Here's how the part is built. I have some questions about the finished solid (model axes, mm). Face numbers are marked on the shaded views. A direction names the side the tool comes from. Give positions to 0.01 mm unless a question says otherwise; leave off trailing zeros. Write each loop counter-clockwise with the first axis right and the second up, starting at its lowest first coordinate (ties: lowest second). Pieces come first, ordered by that corner, then holes. Notation, with made-up numbers: (7, 3) -> (64, 3) arc R24 ccw to (64, 21) -> close; hole circle Ø6 at (27, 52). An arc over 180 degrees is marked (long way). Use CSV: the item, a comma, the result in double quotes. Start each with the question number.
(1) For pin 1 Ø5 at (x, y) = (-24, -3.5) entering from +Z; pin 2 Ø0.9 at (y, z) = (0, 2.5) entering from -X; pin 3 Ø2 at (y, z) = (-2, 11.5) entering from -X, each with a flat end and sliding along its axis, tell me the tip position at first contact or that it passes through.
(2) Suppose I cut it at C-C on z = 11. List the corners of the cut face in (x, y) for me (1 decimal), plus the area to 3 significant figures.
(3) Suppose I cut it at D-D on x = 24.5. List the corners of the cut face in (y, z) for me.
(4) Suppose I cut it at B-B on y = 0. List the corners of the cut face in (x, z) for me, plus the area to 3 significant figures.
(5) I need wall thicknesses on L1, parallel to Z at x = -2, y = -7.75; L2, parallel to Z at x = -29.5, y = 0.75; L3, parallel to Y at x = 24, z = 7.5. Which ranges of each line are inside material? Lowest first, please. Write a range as [from, to].
(6) If we mould it in two halves opening along X, with no side actions, what happens to the marked faces 4, 5, 6 and 7? For each: pulls with the +X half, pulls with the -X half, needs draft (parallel to the pull), parting line crosses it, or undercut.
(7) Which directions (+Z, -Z, +X, -X, +Y, -Y) give clear straight access to the entire face, cutting with the end or side of a thin tool? Please do the marked faces 1, 2 and 3.
(8) Suppose I cut it at A-A on x = -4. List the corners of the cut face in (y, z) for me.
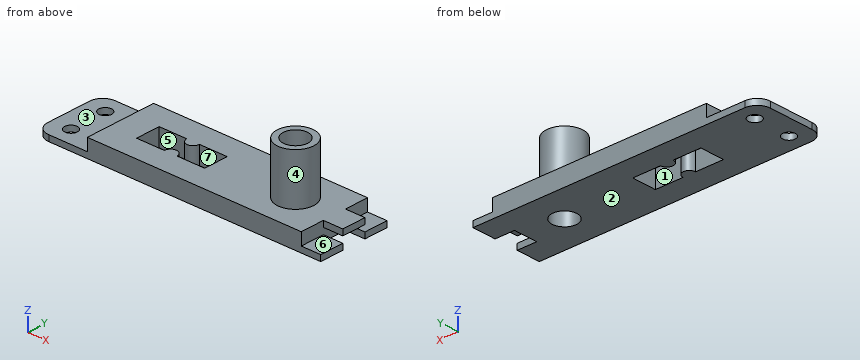
from build123d import *

# Parameters (mm, degrees)
F0_R     = 1.651
F0_R_2   = 4.7625
F0_R_3   = 3.2131
F0_W     = 5.08
F0_H     = 6.223
F1_DEPTH = 1.524
F2_DEPTH = 4.6482
F3_START = 3.1242
F3_DEPTH = 1.524
F4_DEPTH = 16.129


with BuildPart() as f1:
    # F0 (on Top) → F1 (new body)
    with BuildSketch(Plane.XY):
        with BuildLine():
            Line((-23.71344, 0), (-23.71344, 9.3345))
            Line((-23.71344, 9.3345), (-33.782, 9.3345))
            ThreePointArc((-33.782, 9.3345), (-36.2246296649, 8.3227296649), (-37.2364, 5.8801))
            Line((-37.2364, 5.8801), (-37.2364, -5.8801))
            ThreePointArc((-37.2364, -5.8801), (-36.2246296649, -8.3227296649), (-33.782, -9.3345))
            Line((-33.782, -9.3345), (-23.71344, -9.3345))
            Line((-23.71344, -9.3345), (-23.71344, 0))
        make_face()
        with Locations((-32.1564, -4.826)):
            Circle(F0_R, mode=Mode.SUBTRACT)
        with Locations((-32.1564, 4.826)):
            Circle(F0_R, mode=Mode.SUBTRACT)
        Polygon((32.1564, 3.1115), (32.1564, 9.3345), (-23.71344, 9.3345), (-23.71344, 0), (-23.71344, -9.3345), (32.1564, -9.3345), (32.1564, -3.1115), align=None)
        Polygon((-9.3218, -3.18008), (-16.5608, -3.18008), (-16.5608, 3.18008), (-9.3218, 3.18008), (-7.6708, 3.18008), (-6.0198, 3.18008), (1.2192, 3.18008), (1.2192, -3.18008), (-6.0198, -3.18008), (-7.6708, -3.18008), align=None, mode=Mode.SUBTRACT)
        with Locations((21.9964, 0)):
            Circle(F0_R_2, mode=Mode.SUBTRACT)
        with Locations((21.9964, 0)):
            Circle(F0_R_2)
        with Locations((21.9964, 0)):
            Circle(F0_R_3, mode=Mode.SUBTRACT)
        with Locations((34.6964, -6.223)):
            Rectangle(F0_W, F0_H)
        with Locations((34.6964, 6.223)):
            Rectangle(F0_W, F0_H)
        with BuildLine():
            ThreePointArc((-6.0198, -3.18008), (-7.6708, -1.52908), (-9.3218, -3.18008))
            Line((-9.3218, -3.18008), (-7.6708, -3.18008))
            Line((-7.6708, -3.18008), (-6.0198, -3.18008))
        make_face()
        with BuildLine():
            Line((-7.6708, 3.18008), (-9.3218, 3.18008))
            ThreePointArc((-9.3218, 3.18008), (-7.6708, 1.52908), (-6.0198, 3.18008))
            Line((-6.0198, 3.18008), (-7.6708, 3.18008))
        make_face()
    extrude(amount=F1_DEPTH)

    # F0 (on Top) → F2 (join)
    with BuildSketch(Plane.XY):
        Polygon((32.1564, 3.1115), (32.1564, 9.3345), (-23.71344, 9.3345), (-23.71344, 0), (-23.71344, -9.3345), (32.1564, -9.3345), (32.1564, -3.1115), align=None)
        Polygon((-9.3218, -3.18008), (-16.5608, -3.18008), (-16.5608, 3.18008), (-9.3218, 3.18008), (-7.6708, 3.18008), (-6.0198, 3.18008), (1.2192, 3.18008), (1.2192, -3.18008), (-6.0198, -3.18008), (-7.6708, -3.18008), align=None, mode=Mode.SUBTRACT)
        with Locations((21.9964, 0)):
            Circle(F0_R_2, mode=Mode.SUBTRACT)
        with BuildLine():
            ThreePointArc((-6.0198, -3.18008), (-7.6708, -1.52908), (-9.3218, -3.18008))
            Line((-9.3218, -3.18008), (-7.6708, -3.18008))
            Line((-7.6708, -3.18008), (-6.0198, -3.18008))
        make_face()
        with BuildLine():
            Line((-7.6708, 3.18008), (-9.3218, 3.18008))
            ThreePointArc((-9.3218, 3.18008), (-7.6708, 1.52908), (-6.0198, 3.18008))
            Line((-6.0198, 3.18008), (-7.6708, 3.18008))
        make_face()
    extrude(amount=F2_DEPTH)

    # F0 (on Top) → F3 (join)
    with BuildSketch(Plane.XY.offset(F3_START)):
        with Locations((34.6964, 0)):
            Rectangle(F0_W, F0_H)
    extrude(amount=F3_DEPTH)

    # F4 (add): a face of the model
    f4_faces = [f1.faces().sort_by_distance(p)[0] for p in [
        (17.3686038418, 0, 1.524),
    ]]
    extrude(f4_faces, amount=F4_DEPTH)


solid = f1.part
Geometry says:
1,pin 1,"z = 4.65"
1,pin 2,"x = -23.71"
1,pin 3,"x = 17.34"
2,outline,"circle Ø9.5 at (22, 0); hole circle Ø6.4 at (22, 0)"
2,area,"38.8 mm²"
3,outline,"(-9.33, 0) -> (-2.01, 0) -> (-2.01, 17.65) -> (-4.05, 17.65) -> (-4.05, 4.65) -> (-9.33, 4.65) -> close; (2.01, 0) -> (9.33, 0) -> (9.33, 4.65) -> (4.05, 4.65) -> (4.05, 17.65) -> (2.01, 17.65) -> close"
4,outline,"(-37.24, 0) -> (-16.56, 0) -> (-16.56, 4.65) -> (-23.71, 4.65) -> (-23.71, 1.52) -> (-37.24, 1.52) -> close; (1.22, 0) -> (18.78, 0) -> (18.78, 17.65) -> (17.23, 17.65) -> (17.23, 4.65) -> (1.22, 4.65) -> close; (25.21, 0) -> (32.16, 0) -> (32.16, 3.12) -> (37.24, 3.12) -> (37.24, 4.65) -> (26.76, 4.65) -> (26.76, 17.65) -> (25.21, 17.65) -> close"
4,area,"216 mm²"
5,L1,"[0, 4.65]"
5,L2,"[0, 1.52]"
5,L3,"[-4.32, -2.51], [2.51, 4.32]"
6,face 4,"parting line crosses it"
6,face 5,"undercut"
6,face 6,"needs draft"
6,face 7,"undercut"
7,face 1,"+Z, -Z"
7,face 2,"-Z, +X, -X, +Y, -Y"
7,face 3,"+Z, -X, +Y, -Y"
8,outline,"(-9.33, 0) -> (-3.18, 0) -> (-3.18, 4.65) -> (-9.33, 4.65) -> close; (3.18, 0) -> (9.33, 0) -> (9.33, 4.65) -> (3.18, 4.65) -> close"
